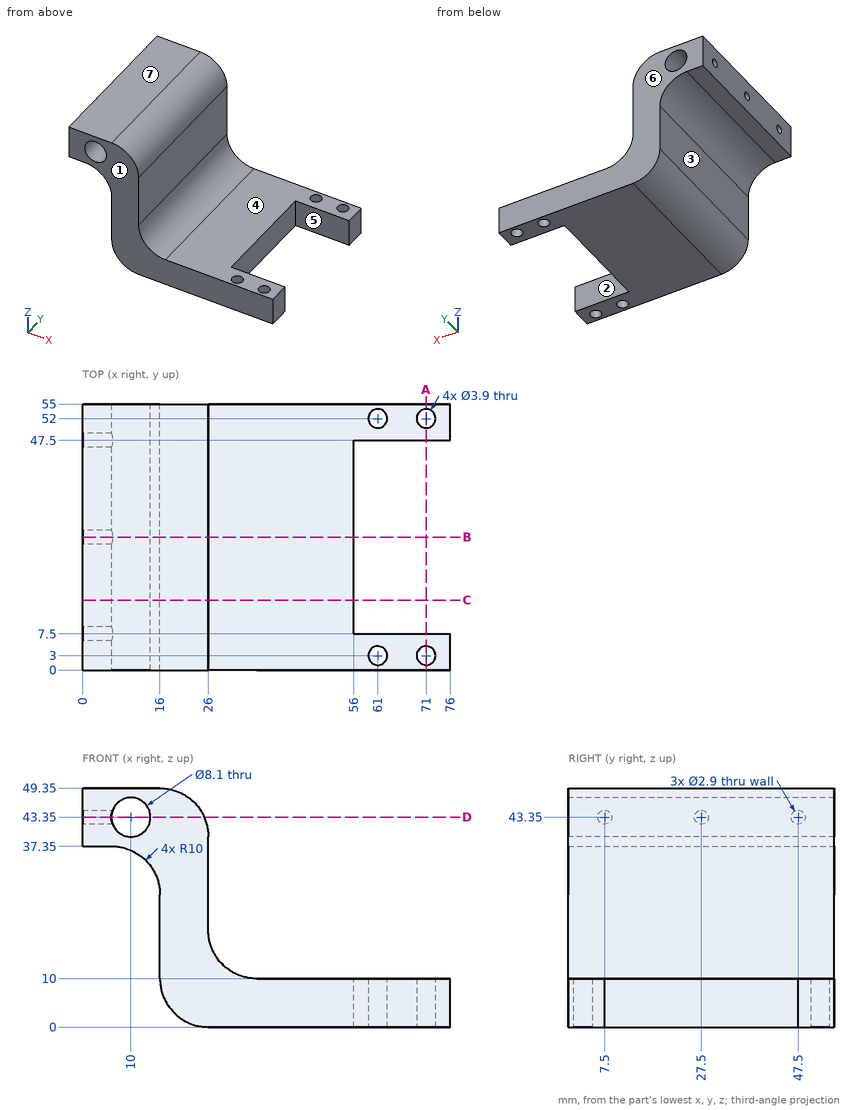
Print and shaded views of the part. All mm, measured from the part's lowest x, y and z. A direction names the side the tool comes from. Coordinates: 2 decimals unless noted, no trailing zeros. Order: outer loops, then holes, each group sorted by start corner. A loop starts at its lowest first (then second) coordinate and runs counter-clockwise, first axis right, second up. Notation, with made-up numbers: M 38.5,58.5 L 57.5,58.5 A14 cw 57.5,76.5 Z; hole C 69.25,34.25 d7. An arc over 180 degrees is marked long. One line per question, with ' | ' between items. Start each with the question number.
Q1. Saw through at D-D (z = 43.35). List the corners of the cut face in (x, y).
Q2. Saw through at A-A (x = 71). List the corners of the cut face in (y, z).
Q3. Flat gauge pins, fed straight in: pin 1 Ø3.5 at (y, z) = (7.5, 43.35) entering from +X; pin 2 Ø13 at (x, z) = (10, 43.35) entering from -Y; pin 3 Ø4 at (y, z) = (16, 22) entering from -X; pin 4 Ø3 at (y, z) = (20, 4) entering from +X. Where does each tip first touch, or does it go through?
Q4. Probe L1, parallel to Y at x = 71, z = 7.25; L2, parallel to Y at x = 4, z = 43; L3, parallel to Z at x = 47, y = 41.5. List the from-to ranges inside material, lowest first. Write a range as from..to.
Q5. Two-plate mould, pull along Y, no slides. Class the marked faces 5, 6 and 7: +Y half, -Y half, draft (parallel to the pull), parting line (faces both ways), or undercut.
Q6. Saw through at C-C (y = 14.5). List the corners of the cut face in (x, z).
Q7. Saw through at B-B (y = 27.5). List the corners of the cut face in (x, z), then the cut area to 3 significant figures.
Q8. 3-axis set-ups, long thin cutter, end or side, ignore diameter. For the marked faces 1, 2, 3 and 4: which of +Z, -Z, +X, -X, +Y, -Y reach the whole face in a straight line?
Check values:
1) outline: M 0,0 L 5.95,0 L 5.95,6.05 L 0,6.05 Z; M 0,8.95 L 5.95,8.95 L 5.95,26.05 L 0,26.05 Z; M 0,28.95 L 5.95,28.95 L 5.95,46.05 L 0,46.05 Z; M 0,48.95 L 5.95,48.95 L 5.95,55 L 0,55 Z; M 14.05,0 L 25.17,0 L 25.17,55 L 14.05,55 Z
2) outline: M 0,0 L 1.05,0 L 1.05,10 L 0,10 Z; M 4.95,0 L 7.5,0 L 7.5,10 L 4.95,10 Z; M 47.5,0 L 50.05,0 L 50.05,10 L 47.5,10 Z; M 53.95,0 L 55,0 L 55,10 L 53.95,10 Z
3) pin 1: stops at x = 25.74 | pin 2: stops at y = 0 | pin 3: stops at x = 16 | pin 4: stops at x = 56
4) L1: y = 0..1.05, 4.95..7.5, 47.5..50.05, 53.95..55 | L2: y = 0..6.09, 8.91..26.09, 28.91..46.09, 48.91..55 | L3: z = 0..10
5) face 5: undercut | face 6: +Y half | face 7: draft
6) outline: M 0,37.35 L 6,37.35 A10 cw 16,27.35 L 16,10 A10 ccw 26,0 L 56,0 L 56,10 L 36,10 A10 cw 26,20 L 26,39.35 A10 ccw 16,49.35 L 0,49.35 Z; hole C 10,43.35 d8.1
7) outline: M 0,37.35 L 6,37.35 A10 cw 16,27.35 L 16,10 A10 ccw 26,0 L 56,0 L 56,10 L 36,10 A10 cw 26,20 L 26,39.35 A10 ccw 16,49.35 L 0,49.35 L 0,44.8 L 6.22,44.8 A4.05 cw long 6.22,41.9 L 0,41.9 Z | area: 916 mm2
8) face 1: +Z, -Z, +X, -X, -Y | face 2: +Z, -Z, +X | face 3: -Z, -X, +Y, -Y | face 4: +Z, +X, +Y, -Y
